Work out the finished part from the listing and answer in its coordinate system (mm). Face numbers are marked on the shaded views. Give positions to 0.01 mm unless a question says otherwise; leave off trailing zeros. Loops run counter-clockwise (first coordinate to the right, second up) from the corner with the lowest first, then second, coordinate; pieces in that order, holes last.
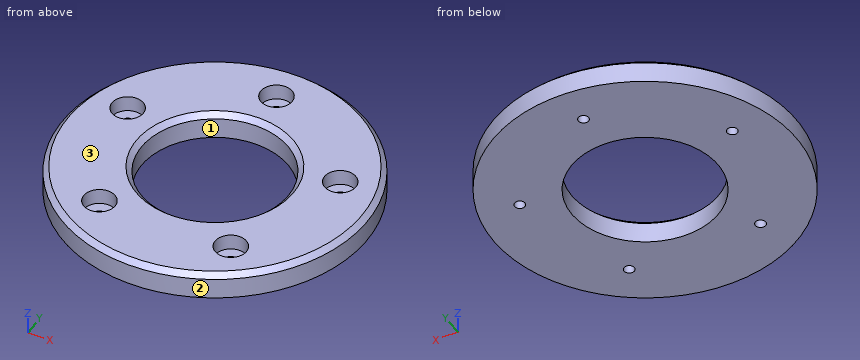
from build123d import *

# Parameters (mm, degrees)
F0_R     = 29
F0_R_2   = 14
F1_DEPTH = 5
F2_R     = 3
F3_DEPTH = 3
F4_R     = 1
F5_DEPTH = 3
F6_SIZE  = 1


with BuildPart() as f1:
    # F0 (on Top) → F1 (new body)
    with BuildSketch(Plane.XY):
        Circle(F0_R)
        Circle(F0_R_2, mode=Mode.SUBTRACT)
    extrude(amount=F1_DEPTH)

    # F2 (on face) → F3 (cut)
    with BuildSketch(Plane.XY.offset(5)):
        with Locations((0, 21.5)):
            Circle(F2_R)
        with Locations((-20.447715, 6.643865)):
            Circle(F2_R)
        with Locations((-12.637383, -17.393865)):
            Circle(F2_R)
        with Locations((12.637383, -17.393865)):
            Circle(F2_R)
        with Locations((20.447715, 6.643865)):
            Circle(F2_R)
    extrude(amount=-F3_DEPTH, mode=Mode.SUBTRACT)

    # F4 (on face) → F5 (cut)
    with BuildSketch(Plane.XY.offset(2)):
        with Locations((0, 21.5)):
            Circle(F4_R)
        with Locations((-20.447715, 6.643865)):
            Circle(F4_R)
        with Locations((-12.637383, -17.393865)):
            Circle(F4_R)
        with Locations((12.637383, -17.393865)):
            Circle(F4_R)
        with Locations((20.447715, 6.643865)):
            Circle(F4_R)
    extrude(amount=-F5_DEPTH, mode=Mode.SUBTRACT)

    # F6
    f6_edges = [f1.edges().sort_by_distance(p)[0] for p in [
        (-29, 0, 5),
        (-14, 0, 5),
    ]]
    chamfer(f6_edges, length=F6_SIZE)


solid = f1.part
Item 1: Flat-ended cylindrical pins translate along their axes: pin 1 Ø2.5 at (x, y) = (-20.45, 6.64) entering from +Z; pin 2 Ø1.6 at (x, y) = (12.64, -17.39) entering from -Z; pin 3 Ø1.5 at (x, z) = (-5.5, 3.5) entering from +Y. Find the tip coordinate at first contact, or state that the pin passes through.
Item 2: Determine the mould class of the marked faces 1, 2 and 3 for opening direction Y: released by +Y, released by -Y, zero draft, split by the parting line, or undercut.
Item 3: Find section A-A, the plane x = 0. Write down the section's boundary in (y, z).
Item 4: Consider line 1 (X direction, y = 6.5, z = 2.3); line 2 (Y direction, x = -11, z = 3.95); line 3 (Y direction, x = -3.5, z = 3.95). Determine where each line is inside the solid, lowest interval first.
Ans:
1. pin 1: stops at z = 2
1. pin 2: passes through
1. pin 3: stops at y = 28.61
2. face 1: undercut
2. face 2: split by the parting line
2. face 3: zero draft
3. outline: (-29, 0) - (-14, 0) - (-14, 4) - (-15, 5) - (-28, 5) - (-29, 4) - close; (14, 0) - (20.5, 0) - (20.5, 2) - (18.5, 2) - (18.5, 5) - (15, 5) - (14, 4) - close; (22.5, 0) - (29, 0) - (29, 4) - (28, 5) - (24.5, 5) - (24.5, 2) - (22.5, 2) - close
4. line 1: x = -28.26 to -23.44, -17.45 to -12.4, 12.4 to 17.45, 23.44 to 28.26
4. line 2: y = -26.83 to -19.91, -14.88 to -8.66, 8.66 to 26.83
4. line 3: y = -28.79 to -13.56, 13.56 to 28.79
